Autodesk Fusion 360 part; units mm, degrees
sketch "Sketch1" plane through (0, 0, 0) normal (0, 0, 1) x (1, 0, 0)
  circle A0 centre (0, 0) radius 31.75
  dimension "d1" = 63.5
extrude "Extrude1" add sketch "Sketch1" along normal blind 50.8
sketch "Sketch2" plane through (0, 0, 50.8) normal (0, 0, 1) x (-1, 0, 0)
  circle A0 centre (0, 0) radius 31.75
  circle A1 centre (0, 0) radius 24.257
  dimension "d4" = 48.514
extrude "Extrude2" cut sketch "Sketch2" against normal blind 25.4 contours A1
fillet "Fillet1" radius 3.175 1 edges at (22.6155, -8.7717, 50.8)
hole "Hole1" at (0, 0, 0) direction (0, 0, 1) diameter 22.631 depth 25 tip angle 118
fillet "Fillet2" radius 1.5875 1 edges at (-29.6014, -11.4813, 0)
fillet "Fillet3" radius 1.5875 1 edges at (-29.6014, -11.4813, 50.8)
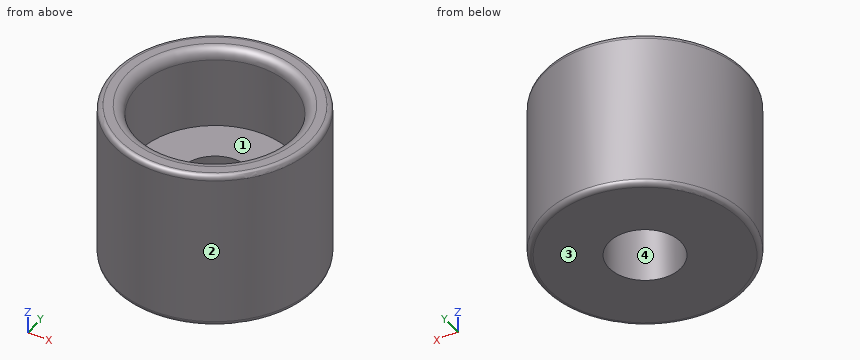
Geometry check sheet. Reference: the model listing, model coordinates, mm. Face numbers are marked on the shaded views. Round coordinates to 2 decimals unless told otherwise and drop trailing zeros. Order: outer loops, then holes, each group sorted by start corner. A loop starts at its lowest first (then second) coordinate and runs counter-clockwise, first axis right, second up. Notation, with made-up numbers: (77.25, 62.25) - (88.25, 62.25) arc R5 ccw to (88.25, 71.25) - close; hole circle Ø4 at (9.25, 59.5). An arc over 180 degrees is marked (long way). Use a Markdown table: item, result. Add a question column.
(1) Material ranges on line 1 along Y through (x, z) = (-0.5, 10); line 2 along Y through (x, z) = (0, 38); line 3 along Z through (x, y) = (3, 15), recorded low to high. Write a range as [from, to].
(2) Depth check by flat-ended pin: pin 1 (10 mm diameter, centred on x = -17.5, z = 42, fed in from -Y); pin 2 (1 mm diameter, centred on x = 25, z = 41, fed in from +Y); pin 3 (6 mm diameter, centred on x = -13.5, z = 43, fed in from -Y). Enter the tip coordinate at first touch or a pass-through.
(3) Release check for a two-part mould opening along X. For the marked faces 1, 2, 3 and 4 record: pulls with the +X half, pulls with the -X half, needs draft (parallel to the pull), parting line crosses it, or undercut.
(4) Sectioned sample at C-C, the plane z = 33.5. Enter the section's corners in (x, y), and give its area (3 significant figures).
(5) Sectioned sample at D-D, the plane z = 21.5. Enter the section's corners in (x, y), and give its area (3 significant figures).
Answers below:
| question | item | result |
|---|---|---|
| 1 | line 1 | [-31.75, -11.3], [11.3, 31.75] |
| 1 | line 2 | [-31.75, -24.26], [24.26, 31.75] |
| 1 | line 3 | [0, 25.4] |
| 2 | pin 1 | y = -29.19 |
| 2 | pin 2 | y = 20.19 |
| 2 | pin 3 | y = -29.96 |
| 3 | face 1 | undercut |
| 3 | face 2 | parting line crosses it |
| 3 | face 3 | needs draft |
| 3 | face 4 | undercut |
| 4 | outline | circle Ø63.5 at (0, 0); hole circle Ø48.51 at (0, 0) |
| 4 | area | 1,320 mm² |
| 5 | outline | circle Ø63.5 at (0, 0); hole circle Ø22.63 at (0, 0) |
| 5 | area | 2,760 mm² |
